from build123d import *

# Parameters (mm, degrees)
F1_DEPTH      = 16
F3_DEPTH      = 8
F3_DEPTH_BACK = 8
F4_W          = 16
F4_H          = 10.4258029827
F5_DEPTH      = 45.4
F7_DEPTH      = 25
F9_START      = -1.5
F9_DEPTH      = 13
F11_START     = -1.5
F11_DEPTH     = 13
F12_W         = 13
F12_H         = 13
F13_DEPTH     = 45.8


# Not quite as in the source:
# - a feature of the source that left no trace in its solid (it failed there, or was rolled back) is left out


with BuildPart() as f1:
    # F0 (on Front) → F1 (new body)
    with BuildSketch(Plane.XZ):
        Polygon((-36.5256857405, 47.6012004175), (0, 0), (36.5256857405, 47.6012004175), align=None)
    extrude(amount=F1_DEPTH)

    # F2 (on Right) → F3 (join, two sides)
    with BuildSketch(Plane.YZ) as f3_sk:
        Polygon((0, 47.6012004175), (0, 0), (47.6012004175, 47.6012004175), align=None)
    extrude(amount=F3_DEPTH)
    extrude(f3_sk.sketch, amount=-F3_DEPTH_BACK)

    # F4 (on face) → F5 (cut)
    with BuildSketch(Plane.XZ.offset(16)):
        with Locations((0, 5.2129014914)):
            Rectangle(F4_W, F4_H)
    extrude(amount=-F5_DEPTH, mode=Mode.SUBTRACT)

    # F6 (on face) → F7 (cut)
    with BuildSketch(Plane.YZ.offset(8)):
        Polygon((37.1753974347, 47.6012004175), (0, 10.4258029827), (10.4258029827, 10.4258029827), (47.6012004175, 47.6012004175), align=None)
    extrude(amount=-F7_DEPTH, mode=Mode.SUBTRACT)

    # F8 (on face) → F9 (cut)
    with BuildSketch(Plane.XZ.offset(16).offset(F9_START)):
        Polygon((-54.3261755364, 73.7560737056), (-17.2410544745, 25.4258029827), (-6.9274610507, 33.3397015598), (-44.0125821126, 81.6699722827), align=None)
        Polygon((6.9274610507, 33.3397015598), (17.2410544745, 25.4258029827), (53.1179434037, 72.181474934), (42.8043499799, 80.0953735111), align=None)
    extrude(amount=-F9_DEPTH, mode=Mode.SUBTRACT)

    # F10 (on face) → F11 (cut)
    with BuildSketch(Plane(origin=(-8, 0, 0), x_dir=(0, -1, 0), z_dir=(-1, 0, 0)).offset(F11_START)):
        Polygon((-16.2450367116, 47.6012004175), (-34.6298130225, 47.6012004175), (-9.8810756809, 22.8524630759), (-0.6886875255, 32.0448512314), align=None)
    extrude(amount=-F11_DEPTH, mode=Mode.SUBTRACT)

    # F12 (on face) → F13 (cut)
    with BuildSketch(Plane(origin=(0, 0, 10.4258029827), x_dir=(1, 0, 0), z_dir=(0, 0, -1))):
        with Locations((0, 8)):
            Rectangle(F12_W, F12_H)
    extrude(amount=-F13_DEPTH, mode=Mode.SUBTRACT)


solid = f1.part
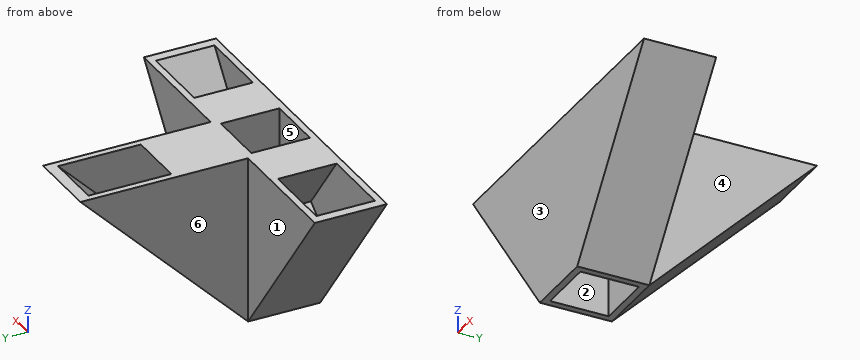
Design review of the part built by this model. Coordinates are the model's own, in mm. Face numbers are marked on the shaded views. A direction names the side the tool comes from. Round coordinates to 2 decimals unless told otherwise and drop trailing zeros. Loops run counter-clockwise (first coordinate to the right, second up) from the corner with the lowest first, then second, coordinate; pieces in that order, holes last. Notation, with made-up numbers: M 66.5,-34.75 L 84.5,-34.75 A15 cw 84.5,-12.75 Z; hole C -35,83.25 d6. An arc over 180 degrees is marked long. Answer as a JSON object with one key per item and string values.
Item 1: Machinability: for the marked faces 4, 5 and 6, which of the approach directions +Z, -Z, +X, -X, +Y, -Y give a long, thin tool a straight path to every point of the face, cutting with its end or side? Answer none if there is none.
Answer sheet:
{"face 4": "+Z, -Z, +X, +Y", "face 5": "+Z, -Z", "face 6": "+Z, -Z, -X, +Y"}
Item 2: We need section A-A on y = -5. Give the boundary of the cut face in (x, z), and give its area (3 significant figures).
Answer sheet:
{"outline": "M -36.53,47.6 L -8,10.43 L -6.5,10.43 L -6.5,47.6 L -17.87,47.6 L -6.93,33.34 L -17.24,25.43 L -34.26,47.6 Z; M 6.5,10.43 L 8,10.43 L 36.53,47.6 L 34.26,47.6 L 17.24,25.43 L 6.93,33.34 L 17.87,47.6 L 6.5,47.6 Z", "area": "575 mm^2"}
Item 3: We need section D-D on x = -21.5. Give the boundary of the cut face in (y, z), and give its area (3 significant figures).
Answer sheet:
{"outline": "M -16,28.02 L 0,28.02 L 0,47.6 L -1.5,47.6 L -1.5,30.98 L -14.5,30.98 L -14.5,47.6 L -16,47.6 Z", "area": "97.2 mm^2"}
Item 4: We need section B-B on z = 16.5. Give the boundary of the cut face in (x, y), and give its area (3 significant figures).
Answer sheet:
{"outline": "M -12.66,-16 L 12.66,-16 L 12.66,0 L 8,0 L 8,6.07 L -8,6.07 L -8,0 L -12.66,0 Z; hole M -6.5,-14.5 L 6.5,-14.5 L 6.5,-1.5 L -6.5,-1.5 Z", "area": "333 mm^2"}
Item 5: We need section C-C on y = 7. Give the boundary of the cut face in (x, z).
Answer sheet:
{"outline": "M -8,17.43 L 8,17.43 L 8,47.6 L -8,47.6 Z; hole M -6.5,25.73 L 6.5,25.73 L 6.5,38.36 L -6.5,38.36 Z"}
Item 6: The part is to be moulded in two halves that separate along Y. For the marked faces 1, 2 and 3, say which applies: pulls with the +Y half, pulls with the -Y half, needs draft (parallel to the pull), parting line crosses it, or undercut.
Answer sheet:
{"face 1": "pulls with the +Y half", "face 2": "undercut", "face 3": "pulls with the -Y half"}
Item 7: Wall thickness on L1, parallel to Y at x = -1.5, z = 38.5; L2, parallel to X at y = 8.5, z = 30.5; L3, parallel to Y at x = 9.5, z = 38.5: over which ranges is each line inside the solid? List them lowest first. Write a range as from..to.
Answer sheet:
{"L1": "y = -16..-14.5, -1.5..7.14, 25.53..28.07", "L2": "x = -8..-6.5, 6.5..8", "L3": "y = -16..0"}
Item 8: Clearance check with flat-ended pins moving along their axes: P1, Ø3, axis at x = 14.5, z = 22, coming from the +Y side; P2, Ø10.5, axis at y = -6.5, z = 27, coming from the -X side; P3, Ø11, axis at y = 27, z = 37.5, coming from the +X side. State where each tip first meets the part, or that it passes through.
Answer sheet:
{"P1": "stops at y = 0", "P2": "stops at x = -24.75", "P3": "stops at x = 8"}
